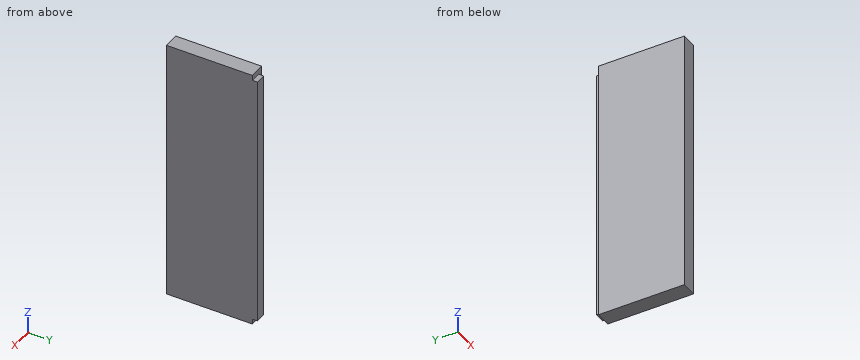
```python
from build123d import *

# Parameters (mm, degrees)
EXTRUDE_1_DEPTH     = 510
SKETCH_2_W          = 10
SKETCH_2_H          = 10
CUT_EXTRUDE_1_DEPTH = 541.023147652


with BuildPart() as part:
    # Эскиз1 → Бобышка-Вытянуть1 (new body)
    with BuildSketch(Plane.XY):
        Polygon((0, 0), (10, 0), (30, 0), (30, 175), (10, 175), (10, 165), (0, 165), align=None)
    extrude(amount=EXTRUDE_1_DEPTH)

    # Эскиз2 → Вырез-Вытянуть1 (cut, through all)
    with BuildSketch(Plane(origin=(30, 0, 0), x_dir=(0, 0, -1), z_dir=(1, 0, 0))):
        with Locations((-5, 170)):
            Rectangle(SKETCH_2_W, SKETCH_2_H)
        with Locations((-505, 170)):
            Rectangle(SKETCH_2_W, SKETCH_2_H)
    extrude(amount=-CUT_EXTRUDE_1_DEPTH, mode=Mode.SUBTRACT)


solid = part.part
```
Could you check a few things on this model? Use its own coordinates, in mm. Round coordinates to 2 decimals unless told otherwise and drop trailing zeros. Write each loop counter-clockwise with the first axis right and the second up, starting at its lowest first coordinate (ties: lowest second). Pieces come first, ordered by that corner, then holes. Notation, with made-up numbers: M -31,16.5 L 2,16.5 A33 cw 2,47.5 Z; hole C 27.5,-30 d4. An arc over 180 degrees is marked long. Answer in a Markdown table with one row per item. Add a question column.
Q1. Imagine slicing it at A-A (z = 93). Please give me the cut outline in (x, y), then the cut area to 3 significant figures.
Q2. Will these pins go through, and if not, where does the flat tip stop? pin 1 Ø11 at (y, z) = (172.5, 304) entering from -X; pin 2 Ø3 at (x, y) = (19, 170.5) entering from +Z; pin 3 Ø1.5 at (x, z) = (9, 142.5) entering from +Y.
Q3. If I drill on line 1 (X direction, y = 167.5, z = 340); line 2 (Y direction, x = 9, z = 118), over which ranges is the centre line in solid material (lowest first)? Write a range as from..to.
Values:
| question | item | result |
|---|---|---|
| 1 | outline | M 0,0 L 30,0 L 30,175 L 10,175 L 10,165 L 0,165 Z |
| 1 | area | 5,150 mm^2 |
| 2 | pin 1 | x = 10 |
| 2 | pin 2 | z = 500 |
| 2 | pin 3 | y = 165 |
| 3 | line 1 | 10..30 |
| 3 | line 2 | 0..165 |
